Can you work these out from the model? Positions are in its coordinate system, mm. Give positions to 0.01 mm unless a question says otherwise; leave off trailing zeros. Loops run counter-clockwise (first coordinate to the right, second up) from the corner with the lowest first, then second, coordinate; pieces in that order, holes last. Notation, with made-up numbers: (5, 26) -> (12, 26) arc R19 ccw to (12, 40) -> close; hole circle Ø3 at (23.25, 46.25). An arc over 180 degrees is marked (long way). Return JSON: item names as keys, results as strings. Group by question number.
Q1. Will these pins go through, and if not, where does the flat tip stop? pin 1 (3 mm diameter, centred on x = -75, y = 25, fed in from +Z); pin 2 (10 mm diameter, centred on x = -44, y = 15, fed in from +Z).
Q2. I need wall thicknesses on line 1 along X through (y, z) = (48, 68); line 2 along X through (y, z) = (54.5, 41); line 3 along Z through (x, y) = (-72.5, 45.5). Which ranges of each line are inside material? Lowest first, please. Write a range as [from, to].
Q3. Suppose I cut it at A-A, the plane x = -82. Please give me the cut outline in (y, z).
Q4. Suppose I cut it at B-B, the plane x = 32. Please give me the cut outline in (y, z).
Q5. Thinking about a two-plate mould opening in Y: for faces 1 (the flat face through (-41, 34, 0)), 2 (the cylindrical face through (-8.06, 31.56, 48.74)), 3 (the flat face through (-41, 0, 31)), which applies, pulls with the +Y half, pulls with the -Y half, needs draft (parallel to the pull), parting line crosses it, or undercut?
Q6. Suppose I cut it at C-C, the plane y = 35.5. Count the separate pieces of the cut face and the enclosed holes in it, and give its area (3 significant figures).
```python
from build123d import *

# Parameters (mm, degrees)
F0_W     = 184.774049
F0_H     = 66.413805
F1_DEPTH = 103.632
F2_SIZE  = 40
F5_D     = 37
F6_D     = 38
F7_R     = 8
F8_R     = 8


with BuildPart() as f1:
    # F0 (on Top) → F1 (new body)
    with BuildSketch(Plane.XY):
        with Locations((-40.078786, 33.206902)):
            Rectangle(F0_W, F0_H)
    extrude(amount=F1_DEPTH)

    # F2
    f2_edges = [f1.edges().sort_by_distance(p)[0] for p in [
        (-40.078785, 0, 103.632),
    ]]
    chamfer(f2_edges, length=F2_SIZE)

    # F5 (through all)
    with Locations(Plane(origin=(0, -31.816, 31.816), x_dir=(1, 0, 0), z_dir=(0, -0.707107, 0.707107))):
        with Locations((-86.328603, 74.946567)):
            Hole(F5_D / 2)

    # F6 (through all)
    with Locations(Plane(origin=(0, -31.816, 31.816), x_dir=(1, 0, 0), z_dir=(0, -0.707107, 0.707107))):
        with Locations((-12.177297, 75.329065)):
            Hole(F6_D / 2)

    # F7
    f7_edges = [f1.edges().sort_by_distance(p)[0] for p in [
        (52.308239, 53.206902, 103.632),
    ]]
    fillet(f7_edges, radius=F7_R)

    # F8
    f8_edges = [f1.edges().sort_by_distance(p)[0] for p in [
        (-132.46581, 53.206902, 103.632),
    ]]
    fillet(f8_edges, radius=F8_R)


solid = f1.part
```
Ans:
{
 "1": {"pin 1": "stops at z = 62.64", "pin 2": "stops at z = 83.63"},
 "2": {"line 1": "x = [-132.47, -103.42], [-69.24, -29.96], [5.6, 52.31]", "line 2": "x = [-132.47, -103.28], [-69.38, -29.5], [5.15, 52.31]", "line 3": "z = [0, 43.11], [77.87, 103.63]"},
 "3": {"outline": "(0, 0) -> (66.41, 0) -> (66.41, 14.14) -> (8.46, 72.09) -> (0, 63.63) -> close; (33.9, 97.53) -> (66.41, 65.01) -> (66.41, 103.63) -> (40, 103.63) -> close"},
 "4": {"outline": "(0, 0) -> (66.41, 0) -> (66.41, 103.63) -> (40, 103.63) -> (0, 63.63) -> close"},
 "5": {"face 1": "needs draft", "face 2": "undercut", "face 3": "pulls with the -Y half"},
 "6": {"separate pieces": "1", "enclosed holes": "2", "area": "15,200 mm^2"}
}
